The model under review builds one solid part; all positions refer to its coordinate system, in mm. A direction names the side the tool comes from. Give positions to 0.01 mm unless a question says otherwise; leave off trailing zeros. Loops run counter-clockwise (first coordinate to the right, second up) from the corner with the lowest first, then second, coordinate; pieces in that order, holes last. Notation, with made-up numbers: (-9.5, 78) - (6.5, 78) arc R8 cw to (6.5, 92) - close; hole circle Ø2 at (57, 24.5). An arc over 180 degrees is marked (long way). Answer as a JSON object with one key per item and string values.
from build123d import *

# Parameters (mm, degrees)
SKETCH1_R           = 66.3575
BOSS_EXTRUDE1_DEPTH = 5.08
CUT_EXTRUDE2_REACH  = 95.981
SKETCH3_R           = 3.900616975
SKETCH3_R_2         = 5.715
SKETCH3_W           = 5.08
SKETCH3_H           = 67.8815


with BuildPart() as part:
    # Sketch1 → Boss-Extrude1 (new body)
    with BuildSketch(Plane.XY):
        Circle(SKETCH1_R)
    extrude(amount=BOSS_EXTRUDE1_DEPTH)

    # Sketch3 → Cut-Extrude2 (cut, up to next)
    with BuildSketch(Plane.XY, mode=Mode.PRIVATE) as cut_extrude2_sk1:
        with Locations((-15.06192248, -40.64)):
            Circle(SKETCH3_R)
    cut_extrude2_tool1 = extrude(cut_extrude2_sk1.sketch, amount=CUT_EXTRUDE2_REACH, mode=Mode.PRIVATE) & part.part
    # Sketch3 → Cut-Extrude2 (cut, up to next)
    with BuildSketch(Plane.XY, mode=Mode.PRIVATE) as cut_extrude2_sk2:
        with Locations((15.41807752, -40.64)):
            Circle(SKETCH3_R)
    cut_extrude2_tool2 = extrude(cut_extrude2_sk2.sketch, amount=CUT_EXTRUDE2_REACH, mode=Mode.PRIVATE) & part.part
    # Sketch3 → Cut-Extrude2 (cut, up to next)
    with BuildSketch(Plane.XY, mode=Mode.PRIVATE) as cut_extrude2_sk3:
        with Locations(Location((15.41807752, 40.64, 0), (0, 0, 180))):
            Circle(SKETCH3_R)
    cut_extrude2_tool3 = extrude(cut_extrude2_sk3.sketch, amount=CUT_EXTRUDE2_REACH, mode=Mode.PRIVATE) & part.part
    # Sketch3 → Cut-Extrude2 (cut, up to next)
    with BuildSketch(Plane.XY, mode=Mode.PRIVATE) as cut_extrude2_sk4:
        with Locations(Location((-15.06192248, 40.64, 0), (0, 0, 180))):
            Circle(SKETCH3_R)
    cut_extrude2_tool4 = extrude(cut_extrude2_sk4.sketch, amount=CUT_EXTRUDE2_REACH, mode=Mode.PRIVATE) & part.part
    # Sketch3 → Cut-Extrude2 (cut, up to next)
    with BuildSketch(Plane.XY, mode=Mode.PRIVATE) as cut_extrude2_sk5:
        with Locations((38.1, -24.368533315)):
            Circle(SKETCH3_R_2)
    cut_extrude2_tool5 = extrude(cut_extrude2_sk5.sketch, amount=CUT_EXTRUDE2_REACH, mode=Mode.PRIVATE) & part.part
    # Sketch3 → Cut-Extrude2 (cut, up to next)
    with BuildSketch(Plane.XY, mode=Mode.PRIVATE) as cut_extrude2_sk6:
        with Locations((0.17807752, -33.91789821)):
            Rectangle(SKETCH3_W, SKETCH3_H)
    cut_extrude2_tool6 = extrude(cut_extrude2_sk6.sketch, amount=CUT_EXTRUDE2_REACH, mode=Mode.PRIVATE) & part.part
    add(cut_extrude2_tool1.solids().sort_by_distance((-15.061922, -40.64, 0))[0], mode=Mode.SUBTRACT)
    add(cut_extrude2_tool2.solids().sort_by_distance((15.418078, -40.64, 0))[0], mode=Mode.SUBTRACT)
    add(cut_extrude2_tool3.solids().sort_by_distance((15.418078, 40.64, 0))[0], mode=Mode.SUBTRACT)
    add(cut_extrude2_tool4.solids().sort_by_distance((-15.061922, 40.64, 0))[0], mode=Mode.SUBTRACT)
    add(cut_extrude2_tool5.solids().sort_by_distance((38.1, -24.368533, 0))[0], mode=Mode.SUBTRACT)
    add(cut_extrude2_tool6.solids().sort_by_distance((0.178078, -33.917898, 0))[0], mode=Mode.SUBTRACT)


solid = part.part
Q1. For faces 5 (the face through (2.718, -34, 3)), 6 (the face through (-1, 1, 5.08)), list the 3-axis set-ups (+Z, -Z, +X, -X, +Y, -Y) from which the entire face can be reached by the end or side of a thin tool; tool diameter is ignored.
Results:
{"face 5": "+Z, -Z, -Y", "face 6": "+Z, +X, -X, +Y, -Y"}
Q2. To check wall thickness, follow probe 1 along Y at (x, z) = (-14.5, 4.1); probe 2 along X at (y, z) = (-40.64, 3.1); probe 3 along X at (y, z) = (-11.5, 2.35). State the ranges of each line that lie inside material, in increasing order. Write a range as [from, to].
Results:
{"probe 1": "y = [-64.75, -44.5], [-36.78, 36.78], [44.5, 64.75]", "probe 2": "x = [-52.46, -18.96], [-11.16, -2.36], [2.72, 11.52], [19.32, 52.46]", "probe 3": "x = [-65.35, -2.36], [2.72, 65.35]"}
Q3. Clearance check with flat-ended pins moving along their axes: pin 1 Ø1.5 at (x, z) = (-39, 0.5) entering from +Y; pin 2 Ø2.5 at (x, z) = (1, 2.5) entering from -Y; pin 3 Ø3 at (y, z) = (-20, 3) entering from +X. State where each tip first meets the part, or that it passes through.
Results:
{"pin 1": "stops at y = 54.22", "pin 2": "stops at y = 0.02", "pin 3": "stops at x = 63.73"}
Q4. Consider section C-C, the plane x = 38.1. State the section outline as (y, z) points, plus the area to 3 significant figures.
Results:
{"outline": "(-54.33, 0) - (-30.08, 0) - (-30.08, 5.08) - (-54.33, 5.08) - close; (-18.65, 0) - (54.33, 0) - (54.33, 5.08) - (-18.65, 5.08) - close", "area": "494 mm^2"}
Q5. Consider section B-B, the plane z = 3.3. State the section outline as (x, y) points (1 decimal), plus the area to 3 significant figures.
Results:
{"outline": "(-2.4, -66.3) - (-2.4, 0) - (2.7, 0) - (2.7, -66.3) arc R66.4 ccw (long way) to start; hole circle Ø7.8 at (-15.1, -40.6); hole circle Ø7.8 at (-15.1, 40.6); hole circle Ø7.8 at (15.4, -40.6); hole circle Ø7.8 at (15.4, 40.6); hole circle Ø11.4 at (38.1, -24.4)", "area": "13,200 mm^2"}
Q6. The part is to be moulded in two halves that separate along Y. For faces 1 (the face through (-14.22, 44.45, 2.5)), 2 (the face through (0, 0.023, 3)), 3 (the face through (-2.362, -34, 3)), 4 (the face through (37.36, -18.7, 2.5)), say which applies: +Y half, -Y half, draft (parallel to the pull), parting line (faces both ways), or undercut.
Results:
{"face 1": "undercut", "face 2": "-Y half", "face 3": "draft", "face 4": "undercut"}
Q7. Consider section A-A, the plane y = -8.5. State the section outline as (x, z) points.
Results:
{"outline": "(-65.81, 0) - (-2.36, 0) - (-2.36, 5.08) - (-65.81, 5.08) - close; (2.72, 0) - (65.81, 0) - (65.81, 5.08) - (2.72, 5.08) - close"}
Q8. Consider section D-D, the plane y = 40.64. State the section outline as (x, z) points, plus the area to 3 significant figures.
Results:
{"outline": "(-52.46, 0) - (-18.96, 0) - (-18.96, 5.08) - (-52.46, 5.08) - close; (-11.16, 0) - (11.52, 0) - (11.52, 5.08) - (-11.16, 5.08) - close; (19.32, 0) - (52.46, 0) - (52.46, 5.08) - (19.32, 5.08) - close", "area": "454 mm^2"}
